Can you work these out from the model? Positions are in its coordinate system, mm. Face numbers are marked on the shaded views. A direction names the side the tool comes from. Round coordinates to 2 decimals unless told otherwise and drop trailing zeros. Loops run counter-clockwise (first coordinate to the right, second up) from the corner with the lowest first, then second, coordinate; pieces in that order, holes last. Notation, with made-up numbers: (73.5, 80) -> (118.5, 80) arc R10 ccw to (118.5, 95) -> close; hole circle Ø4 at (6, -0.5). An arc over 180 degrees is marked (long way). Write item = value, one per line.
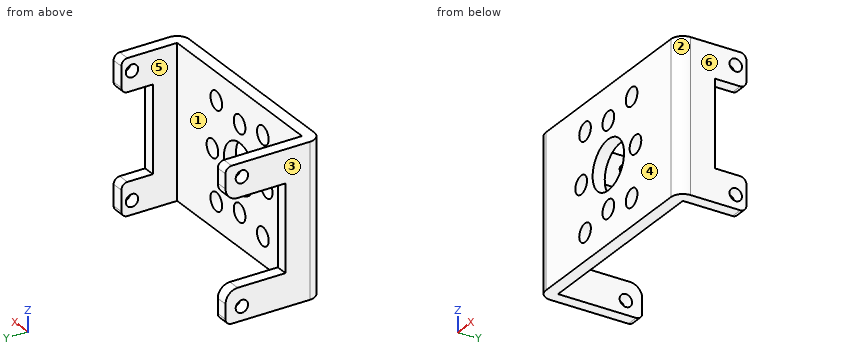
from build123d import *

# Parameters (mm, degrees)
EXTRUDE_1_DEPTH     = 25
SKETCH_2_R          = 1.025
CUT_EXTRUDE_1_DEPTH = 50
FILLET_1_R          = 1
SKETCH_3_R          = 1.025
CUT_EXTRUDE_2_DEPTH = 6
SKETCH_4_R          = 4.05
SKETCH_4_R_2        = 1.5
CUT_EXTRUDE_3_DEPTH = 10


with BuildPart() as part:
    # 草图1 → 凸台-拉伸1 (new body)
    with BuildSketch(Plane.XY):
        with BuildLine():
            Line((2, 0), (34.2, 0))
            ThreePointArc((34.2, 0), (35.614213562, 0.585786438), (36.2, 2))
            Line((36.2, 2), (36.2, 11.2))
            Line((36.2, 11.2), (34.2, 11.2))
            Line((34.2, 11.2), (34.2, 2))
            Line((34.2, 2), (2, 2))
            Line((2, 2), (2, 15.9))
            Line((2, 15.9), (0, 15.9))
            Line((0, 15.9), (0, 2))
            ThreePointArc((0, 2), (0.585786438, 0.585786438), (2, 0))
        make_face()
    extrude(amount=EXTRUDE_1_DEPTH)

    # 草图2 → 切除-拉伸1 (cut)
    with BuildSketch(Plane.ZY):
        with BuildLine():
            Line((0, 15.9), (0, 14.9))
            ThreePointArc((0, 14.9), (0.292893219, 15.607106781), (1, 15.9))
            Line((1, 15.9), (0, 15.9))
        make_face()
        with Locations((2.25, 13.2)):
            Circle(SKETCH_2_R)
        with BuildLine():
            Line((21.6, 15.9), (3.4, 15.9))
            ThreePointArc((3.4, 15.9), (4.814213562, 15.314213562), (5.4, 13.9))
            Line((5.4, 13.9), (5.4, 6))
            Line((5.4, 6), (19.6, 6))
            Line((19.6, 6), (19.6, 13.9))
            ThreePointArc((19.6, 13.9), (20.185786438, 15.314213562), (21.6, 15.9))
        make_face()
        with Locations((22.75, 13.2)):
            Circle(SKETCH_2_R)
        with BuildLine():
            Line((25, 15.9), (24, 15.9))
            ThreePointArc((24, 15.9), (24.707106781, 15.607106781), (25, 14.9))
            Line((25, 14.9), (25, 15.9))
        make_face()
    extrude(amount=-CUT_EXTRUDE_1_DEPTH, mode=Mode.SUBTRACT)

    # 圆角1
    fillet_1_edges = [part.edges().sort_by_distance(p)[0] for p in [
        (35.2, 11.2, 0),
        (35.2, 11.2, 25),
        (35.2, 11.2, 19.6),
        (35.2, 11.2, 5.4),
    ]]
    fillet(fillet_1_edges, radius=FILLET_1_R)

    # 草图3 → 切除-拉伸2 (cut)
    with BuildSketch(Plane(origin=(36.2, 0, 0), x_dir=(0, 0, -1), z_dir=(1, 0, 0))):
        with Locations((-22.75, 9.45)):
            Circle(SKETCH_3_R)
        with Locations((-2.25, 9.45)):
            Circle(SKETCH_3_R)
    extrude(amount=-CUT_EXTRUDE_2_DEPTH, mode=Mode.SUBTRACT)

    # 草图4 → 切除-拉伸3 (cut)
    with BuildSketch(Plane(origin=(0, 2, 0), x_dir=(1, 0, 0), z_dir=(0, 1, 0))):
        with Locations(Location((18.1, -12.5, 0), (0, 0, 270))):
            Circle(SKETCH_4_R)
        with Locations(Location((18.1, -5.5, 0), (0, 0, 270))):
            Circle(SKETCH_4_R_2)
        with Locations(Location((25.1, -12.5, 0), (0, 0, 270))):
            Circle(SKETCH_4_R_2)
        with Locations(Location((18.1, -19.5, 0), (0, 0, 270))):
            Circle(SKETCH_4_R_2)
        with Locations(Location((11.1, -12.5, 0), (0, 0, 270))):
            Circle(SKETCH_4_R_2)
        with Locations(Location((12.1, -4.5, 0), (0, 0, 270))):
            Circle(SKETCH_4_R_2)
        with Locations(Location((24.1, -4.5, 0), (0, 0, 270))):
            Circle(SKETCH_4_R_2)
        with Locations(Location((24.1, -20.5, 0), (0, 0, 270))):
            Circle(SKETCH_4_R_2)
        with Locations(Location((12.1, -20.5, 0), (0, 0, 270))):
            Circle(SKETCH_4_R_2)
    extrude(amount=-CUT_EXTRUDE_3_DEPTH, mode=Mode.SUBTRACT)


solid = part.part
1. For the marked faces 5 and 6, which set-ups out of +Z, -Z, +X, -X, +Y, -Y let a thin tool reach every point of the face, with its end or its side?
Entries:
face_5 = +Z, -Z, +Y
face_6 = +Z, -Z, +X, +Y, -Y
2. We'd pull the mould along X, two halves only. Please class the marked faces 1, 2, 3 and 4: released by +X, released by -X, zero draft, split by the parting line, or undercut.
Entries:
face_1 = undercut
face_2 = released by +X
face_3 = released by -X
face_4 = zero draft
3. Suppose I cut it at D-D, the plane y = 4.5. List the corners of the cut face in (x, z) for me.
Entries:
outline = (0, 0) -> (2, 0) -> (2, 25) -> (0, 25) -> close; (34.2, 0) -> (36.2, 0) -> (36.2, 25) -> (34.2, 25) -> close
4. Suppose I cut it at A-A, the plane y = 13.2. List the corners of the cut face in (x, z) for me (3 decimals), and give its area (3 significant figures).
Entries:
outline = (0, 0) -> (2, 0) -> (2, 1.225) -> (0, 1.225) -> close; (0, 3.275) -> (2, 3.275) -> (2, 5.4) -> (0, 5.4) -> close; (0, 19.6) -> (2, 19.6) -> (2, 21.725) -> (0, 21.725) -> close; (0, 23.775) -> (2, 23.775) -> (2, 25) -> (0, 25) -> close
area = 13.4 mm²
5. Suppose I cut it at B-B, the plane z = 2.25. List the corners of the cut face in (x, y) for me (3 decimals), and give its area (3 significant figures).
Entries:
outline = (0, 2) arc R2 ccw to (2, 0) -> (34.2, 0) arc R2 ccw to (36.2, 2) -> (36.2, 8.425) -> (34.2, 8.425) -> (34.2, 2) -> (2, 2) -> (2, 12.175) -> (0, 12.175) -> close; (0, 14.225) -> (2, 14.225) -> (2, 15.9) -> (0, 15.9) -> close; (34.2, 10.475) -> (36.2, 10.475) -> (36.2, 11.2) -> (34.2, 11.2) -> close
area = 109 mm²
6. Suppose I cut it at C-C, the plane x = 18.1. List the corners of the cut face in (y, z) for me.
Entries:
outline = (0, 0) -> (2, 0) -> (2, 4) -> (0, 4) -> close; (0, 7) -> (2, 7) -> (2, 8.45) -> (0, 8.45) -> close; (0, 16.55) -> (2, 16.55) -> (2, 18) -> (0, 18) -> close; (0, 21) -> (2, 21) -> (2, 25) -> (0, 25) -> close
7. I need wall thicknesses on line 1 (X direction, y = 4.5, z = 14.5); line 2 (X direction, y = 0.8, z = 12.5); line 3 (X direction, y = 1.15, z = 12.5). Which ranges of each line are inside material? Lowest first, please. Write a range as [from, to].
Entries:
line_1 = [0, 2], [34.2, 36.2]
line_2 = [0.4, 9.6], [12.6, 14.05], [22.15, 23.6], [26.6, 35.8]
line_3 = [0.19, 9.6], [12.6, 14.05], [22.15, 23.6], [26.6, 36.01]
8. I'm going to push flat-ended pins straight in: pin 1 (2 mm diameter, centred on x = 24, z = 16, fed in from -Y); pin 2 (6.5 mm diameter, centred on x = 18.1, z = 12.5, fed in from +Y); pin 3 (1.6 mm diameter, centred on x = 35, z = 11, fed in from +Y); pin 4 (4 mm diameter, centred on x = 25.1, z = 12.5, fed in from +Y). Where does each tip first touch, or does it pass through?
Entries:
pin_1 = 0
pin_2 = through
pin_3 = 6
pin_4 = 2
